from build123d import *

# Parameters (mm, degrees)
SKETCH1_W                 = 113.538
SKETCH1_H                 = 88.138
EXTRUDE1_DEPTH            = 6.35
F_8_CLEARANCE_HOLE1_D     = 4.0386
F_8_CLEARANCE_HOLE1_DEPTH = 6.35
FILLET2_R                 = 3.175


with BuildPart() as part:
    # Sketch1 → Extrude1 (new body)
    with BuildSketch(Plane.XY):
        Rectangle(SKETCH1_W, SKETCH1_H)
    extrude(amount=EXTRUDE1_DEPTH)

    # #8 Clearance Hole1
    with Locations(Plane(origin=(-52.3875, 39.6875, 6.35), x_dir=(1, 0, 0), z_dir=(0, 0, 1))):
        with Locations((0, 0), (104.775, 0), (104.775, -79.375), (0, -79.375)):
            Hole(F_8_CLEARANCE_HOLE1_D / 2, depth=F_8_CLEARANCE_HOLE1_DEPTH)

    # Fillet2
    fillet2_edges = [part.edges().sort_by_distance(p)[0] for p in [
        (-56.769, 44.069, 3.175),
        (56.769, 44.069, 3.175),
        (56.769, -44.069, 3.175),
        (-56.769, -44.069, 3.175),
    ]]
    fillet(fillet2_edges, radius=FILLET2_R)


solid = part.part
Input: part model. Units: mm. Frame: model coordinates. Coordinates: 2 decimals unless noted, no trailing zeros. Answer in a Markdown table with one row per item.
(1) Material intervals for line 1 (X direction, y = 38, z = 3.25), sorted ascending. Write a range as [from, to].
Numbers:
| item | result |
|---|---|
| line 1 | x = [-56.77, -53.5], [-51.28, 51.28], [53.5, 56.77] |
(2) Draft query along X for faces 1 (the cylindrical face through (-51.95, -41.66, 3.13)), 2 (the flat face through (-1, 44.069, 3)), 3 (the flat face through (-56.769, -1, 3)). Return one class per face: pulls with the +X half, pulls with the -X half, needs draft (parallel to the pull), parting line crosses it, or undercut.
Numbers:
| item | result |
|---|---|
| face 1 | undercut |
| face 2 | needs draft |
| face 3 | pulls with the -X half |
(3) Contact query for flat-ended pins moving along their axis: pin 1 Ø6.5 at (x, y) = (52.39, -39.69) entering from -Z; pin 2 Ø3.5 at (x, y) = (-52.39, -39.69) entering from +Z (3 decimals). Output: stop coordinate, or through.
Numbers:
| item | result |
|---|---|
| pin 1 | stops at z = 0 |
| pin 2 | passes through |
